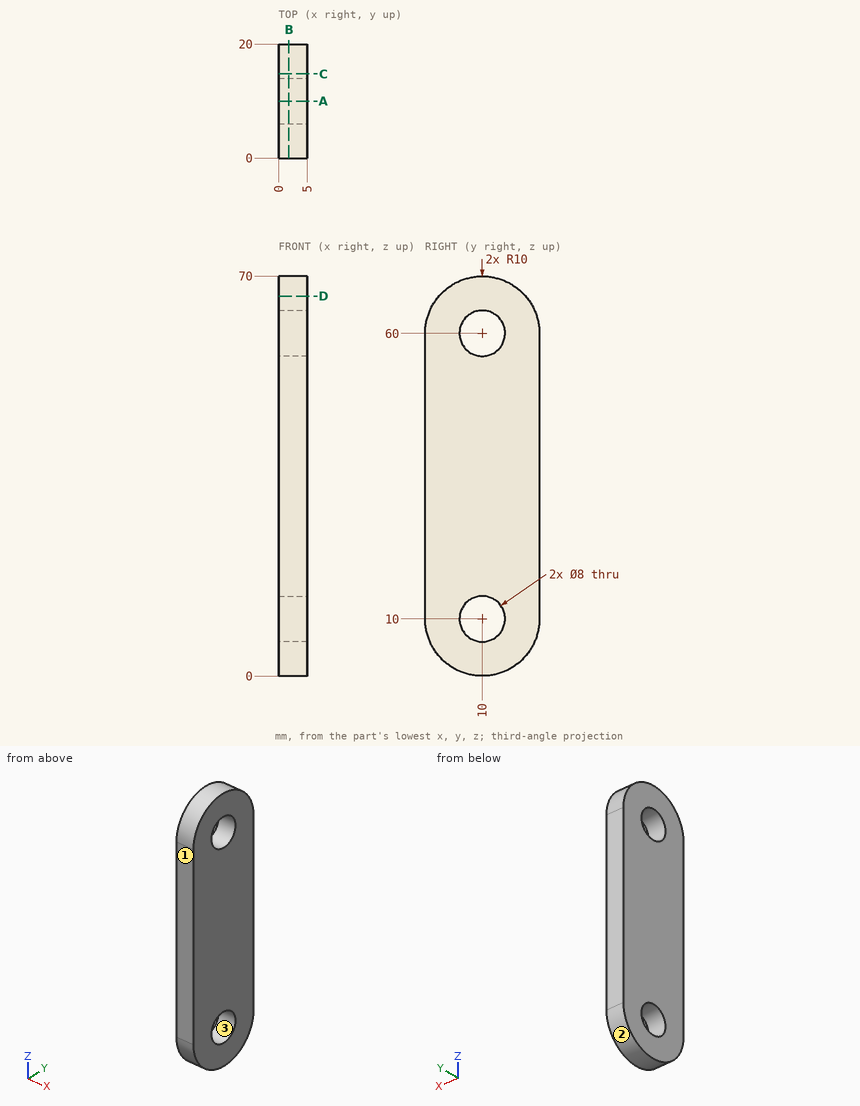
Geometry check sheet. Reference: drawing and pictorial views, mm from the part's lowest x, y, z. Round coordinates to 2 decimals unless told otherwise and drop trailing zeros. Order: outer loops, then holes, each group sorted by start corner. A loop starts at its lowest first (then second) coordinate and runs counter-clockwise, first axis right, second up. Notation, with made-up numbers: (73, 74) - (80, 74) arc R18 ccw to (80, 85) - close; hole circle Ø3 at (80, 9). An arc over 180 degrees is marked (long way). Use a Markdown table: item, result. Add a question column.
1) Section check A-A (y = 10). Record the cut outline in (x, z).
2) Thickness scan on line 1 along Y through (x, z) = (1.55, 10); line 2 along Z through (x, y) = (1.75, 11); line 3 along Z through (x, y) = (3.85, 13.25). Record the ranges inside material, lowest first.
3) Section check D-D (z = 66.5). Record the cut outline in (x, y).
4) Mould release check, pull along Y, two halves, no side actions. Record for the marked faces 1, 2 and 3: released by +Y, released by -Y, zero draft, split by the parting line, or undercut.
5) Section check C-C (y = 14.75). Record the cut outline in (x, z), then the cut area to 3 significant figures.
6) Section check B-B (x = 1.8). Record the cut outline in (y, z).
7) Gauge pin test, flat end, axial feed: P1, Ø3, axis at y = 3, z = 24, coming from the -X side. Record the tip position at first contact, or that the pin passes through.
Established:
| question | item | result |
|---|---|---|
| 1 | outline | (0, 0) - (5, 0) - (5, 6) - (0, 6) - close; (0, 14) - (5, 14) - (5, 56) - (0, 56) - close; (0, 64) - (5, 64) - (5, 70) - (0, 70) - close |
| 2 | line 1 | 0 to 6, 14 to 20 |
| 2 | line 2 | 0.05 to 6.13, 13.87 to 56.13, 63.87 to 69.95 |
| 2 | line 3 | 0.54 to 7.67, 12.33 to 57.67, 62.33 to 69.46 |
| 3 | outline | (0, 2.4) - (5, 2.4) - (5, 17.6) - (0, 17.6) - close |
| 4 | face 1 | released by -Y |
| 4 | face 2 | split by the parting line |
| 4 | face 3 | undercut |
| 5 | outline | (0, 1.2) - (5, 1.2) - (5, 68.8) - (0, 68.8) - close |
| 5 | area | 338 mm2 |
| 6 | outline | (0, 10) arc R10 ccw to (20, 10) - (20, 60) arc R10 ccw to (0, 60) - close; hole circle Ø8 at (10, 10); hole circle Ø8 at (10, 60) |
| 7 | P1 | x = 0 |
